from build123d import *

# Parameters (mm, degrees)
PAD_DEPTH            = 10
SKETCH003_R          = 1.6
POCKET_DEPTH         = 0.001
POCKET_DEPTH_BACK    = 10.001
SKETCH006_W          = 6
SKETCH006_H          = 5
PAD001_DEPTH         = 1
PAD001_TAPER         = 45
SKETCH_R             = 1.6
POCKET004_DEPTH      = 11.501
POCKET004_DEPTH_BACK = 0.001
FILLET_R             = 1.5
CHAMFER_SIZE         = 0.4


with BuildPart() as part:
    # Sketch001 → Pad (new body)
    with BuildSketch(Plane.XY):
        Polygon((-3.5, 18), (-3.5, 0), (-3.5, -18), (8, -18), (8, 18), align=None)
    extrude(amount=PAD_DEPTH)

    # Sketch003 → Pocket (cut, two sides)
    with BuildSketch(Plane.XY) as pocket_sk:
        Circle(SKETCH003_R)
    extrude(amount=-POCKET_DEPTH, mode=Mode.SUBTRACT)
    extrude(pocket_sk.sketch, amount=POCKET_DEPTH_BACK, mode=Mode.SUBTRACT)

    # Sketch006 (on Face5 of Pocket) → Pad001 (join)
    with BuildSketch(Plane.XY.offset(10)):
        with Locations((0, 10.5)):
            Rectangle(SKETCH006_W, SKETCH006_H)
        with Locations((0, -10.5)):
            Rectangle(SKETCH006_W, SKETCH006_H)
    extrude(amount=PAD001_DEPTH, taper=PAD001_TAPER)

    # Sketch (on Face2 of Pad001) → Pocket004 (cut, two sides)
    with BuildSketch(Plane(origin=(-3.5, 0, 0), x_dir=(0, -1, 0), z_dir=(-1, 0, 0))) as pocket004_sk:
        with Locations((-12.5, 4)):
            Circle(SKETCH_R)
        with Locations((12.5, 4)):
            Circle(SKETCH_R)
    extrude(amount=-POCKET004_DEPTH, mode=Mode.SUBTRACT)
    extrude(pocket004_sk.sketch, amount=POCKET004_DEPTH_BACK, mode=Mode.SUBTRACT)

    # Fillet
    fillet_edges = [part.edges().sort_by_distance(p)[0] for p in [
        (-3.5, -18, 5),
        (8, -18, 5),
        (-3.5, 18, 5),
        (8, 18, 5),
    ]]
    fillet(fillet_edges, radius=FILLET_R)

    # Chamfer
    chamfer_edges = [part.edges().sort_by_distance(p)[0] for p in [
        (-3.5, 0, 0),
        (-3.06066, 17.56066, 0),
        (-3.06066, -17.56066, 0),
        (2.25, 18, 0),
        (2.25, -18, 0),
        (7.56066, 17.56066, 0),
        (7.56066, -17.56066, 0),
        (8, 0, 0),
        (-1.6, 0, 0),
        (2.25, 18, 10),
        (-1.6, 0, 10),
    ]]
    chamfer(chamfer_edges, length=CHAMFER_SIZE)


solid = part.part
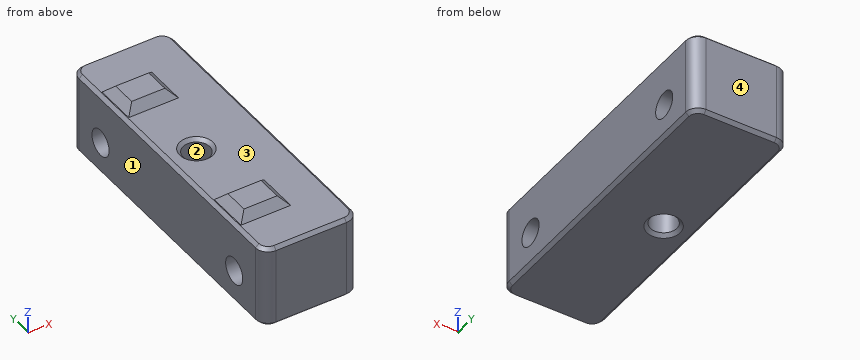
Here's how the part is built. I have some questions about the finished solid (model axes, mm). Face numbers are marked on the shaded views. Give positions to 0.01 mm unless a question says otherwise; leave off trailing zeros. Order: outer loops, then holes, each group sorted by start corner. A loop starts at its lowest first (then second) coordinate and runs counter-clockwise, first axis right, second up. Notation, with made-up numbers: (64.5, 59) -> (123.5, 59) arc R8 ccw to (123.5, 66) -> close; hole circle Ø3 at (4, -8.75). An arc over 180 degrees is marked (long way). One line per item, written item: value. Start each with the question number.
1. I need wall thicknesses on probe 1 along X at (y, z) = (0, 4.75); probe 2 along Y at (x, z) = (0, 7.25); probe 3 along Y at (x, z) = (6.5, 3.5). Which ranges of each line are inside material? Lowest first, please. Write a range as from..to.
2. Imagine slicing it at B-B, the plane x = 0. List the corners of the cut face in (y, z) for me, plus the area to 3 significant figures.
3. Imagine slicing it at C-C, the plane y = -9.5. List the corners of the cut face in (x, z) for me, plus the area to 3 significant figures.
4. We'd pull the mould along Y, two halves only. Please class the marked faces 1, 2, 3 and 4: released by +Y, released by -Y, zero draft, split by the parting line, or undercut.
5. Imagine slicing it at A-A, the plane y = 0. List the corners of the cut face in (x, z) for me, plus the area to 3 significant figures.
6. Will these pins go through, and if not, where does the flat tip stop? pin 1 Ø3 at (x, y) = (0, 0) entering from +Z; pin 2 Ø3.5 at (y, z) = (-12.5, 4) entering from +X.
7. Imagine slicing it at D-D, the plane y = 12.5. List the corners of the cut face in (x, z) for me.
Values follow:
1. probe 1: x = -3.5..-1.6, 1.6..8
1. probe 2: y = -18..-1.6, 1.6..18
1. probe 3: y = -18..-14.02, -10.98..10.98, 14.02..18
2. outline: (-18, 0.4) -> (-17.6, 0) -> (-2, 0) -> (-1.6, 0.4) -> (-1.6, 9.6) -> (-2, 10) -> (-8, 10) -> (-9, 11) -> (-12, 11) -> (-13, 10) -> (-17.6, 10) -> (-18, 9.6) -> close; (1.6, 0.4) -> (2, 0) -> (17.6, 0) -> (18, 0.4) -> (18, 9.6) -> (17.6, 10) -> (13, 10) -> (12, 11) -> (9, 11) -> (8, 10) -> (2, 10) -> (1.6, 9.6) -> close; hole circle Ø3.2 at (-12.5, 4); hole circle Ø3.2 at (12.5, 4)
2. area: 319 mm2
3. outline: (-3.5, 0.4) -> (-3.1, 0) -> (7.6, 0) -> (8, 0.4) -> (8, 9.6) -> (7.6, 10) -> (3, 10) -> (2, 11) -> (-2, 11) -> (-3, 10) -> (-3.1, 10) -> (-3.5, 9.6) -> close
3. area: 120 mm2
4. face 1: zero draft
4. face 2: undercut
4. face 3: undercut
4. face 4: released by +Y
5. outline: (-3.5, 0.4) -> (-3.1, 0) -> (-2, 0) -> (-1.6, 0.4) -> (-1.6, 9.6) -> (-2, 10) -> (-3.1, 10) -> (-3.5, 9.6) -> close; (1.6, 0.4) -> (2, 0) -> (7.6, 0) -> (8, 0.4) -> (8, 9.6) -> (7.6, 10) -> (2, 10) -> (1.6, 9.6) -> close
5. area: 82.4 mm2
6. pin 1: passes through
6. pin 2: stops at x = 8
7. outline: (-3.5, 0.4) -> (-3.1, 0) -> (7.6, 0) -> (8, 0.4) -> (8, 2.4) -> (-3.5, 2.4) -> close; (-3.5, 5.6) -> (8, 5.6) -> (8, 9.6) -> (7.6, 10) -> (3, 10) -> (2.5, 10.5) -> (-2.5, 10.5) -> (-3, 10) -> (-3.1, 10) -> (-3.5, 9.6) -> close
